Input: part model. Units: mm. Frame: model coordinates. Give positions to 0.01 mm unless a question says otherwise; leave off trailing zeros. Loops run counter-clockwise (first coordinate to the right, second up) from the corner with the lowest first, then second, coordinate; pieces in that order, holes last. Notation, with made-up numbers: (20.25, -36.75) - (29.25, -36.75) arc R20 ccw to (29.25, -29.75) - close; hole circle Ø11 at (50.25, 43). An arc over 180 degrees is marked (long way). Answer as a JSON object with one key per item and string values. Group by question number.
(1) Pin query (flat end, axial travel): P1, Ø4.5, axis at x = 60.325, z = -30.48, coming from the -Y side. Return the tip coordinate at first contact, or that it passes through.
(2) Section query D-D (z = 25.4). Return loops of the section in (x, y) (1 decimal), plus the area to 3 significant figures.
(3) Section query B-B (x = 0). Return loops of the section in (y, z), plus the area to 3 significant figures.
(4) Section query A-A (z = -30.48). Return loops of the section in (x, y) (3 decimals), plus the area to 3 significant figures.
(5) Mould query, pull axis Z, two halves, no side actions, for faces 1 (the flat face through (1, 2, 35.56)), 2 (the cylindrical face through (57.845, 2.129, -31.031)), 3 (the flat face through (66.675, 2, 0)). Classes: +Z half, -Z half, draft (parallel to the pull), parting line (faces both ways), or undercut.
(6) Section query C-C (z = 0). Return loops of the section in (x, y) (3 decimals), plus the area to 3 significant figures.
(7) Material intervals for L1, parallel to X at y = 3.15, z = 30.48 (3 decimals); L2, parallel to X at y = 3.6, z = -0.5 (3 decimals); L3, parallel to X at y = 1.25, z = 24.5 (3 decimals), sorted ascending.
```python
from build123d import *

# Parameters (mm, degrees)
SKETCH1_R           = 29.21
SKETCH1_R_2         = 2.2225
SKETCH1_R_3         = 2.54
BOSS_EXTRUDE1_DEPTH = 4.318


with BuildPart() as part:
    # Sketch1 → Boss-Extrude1 (new body)
    with BuildSketch(Plane(origin=(0, 0, 0), x_dir=(1, 0, 0), z_dir=(0, 1, 0))):
        Polygon((0, 35.56), (66.675, 35.56), (66.675, -35.56), (-66.675, -35.56), (-66.675, 35.56), align=None)
        with Locations(Location((0, 0, 0), (0, 0, 270))):
            Circle(SKETCH1_R, mode=Mode.SUBTRACT)
        with Locations(Location((25.4, -25.4, 0), (0, 0, 270))):
            Circle(SKETCH1_R_2, mode=Mode.SUBTRACT)
        with Locations(Location((25.4, 25.4, 0), (0, 0, 270))):
            Circle(SKETCH1_R_2, mode=Mode.SUBTRACT)
        with Locations(Location((-25.4, 25.4, 0), (0, 0, 270))):
            Circle(SKETCH1_R_2, mode=Mode.SUBTRACT)
        with Locations(Location((-25.4, -25.4, 0), (0, 0, 270))):
            Circle(SKETCH1_R_2, mode=Mode.SUBTRACT)
        with Locations(Location((-60.325, -30.48, 0), (0, 0, 270))):
            Circle(SKETCH1_R_3, mode=Mode.SUBTRACT)
        with Locations(Location((-60.325, 30.48, 0), (0, 0, 270))):
            Circle(SKETCH1_R_3, mode=Mode.SUBTRACT)
        with Locations(Location((60.325, 30.48, 0), (0, 0, 270))):
            Circle(SKETCH1_R_3, mode=Mode.SUBTRACT)
        with Locations(Location((60.325, -30.48, 0), (0, 0, 270))):
            Circle(SKETCH1_R_3, mode=Mode.SUBTRACT)
    extrude(amount=BOSS_EXTRUDE1_DEPTH)


solid = part.part
```
Recorded:
{
 "1": {"P1": "passes through"},
 "2": {"outline": "(-66.7, 0) - (-27.6, 0) - (-27.6, 4.3) - (-66.7, 4.3) - close; (-23.2, 0) - (-14.4, 0) - (-14.4, 4.3) - (-23.2, 4.3) - close; (14.4, 0) - (23.2, 0) - (23.2, 4.3) - (14.4, 4.3) - close; (27.6, 0) - (66.7, 0) - (66.7, 4.3) - (27.6, 4.3) - close", "area": "413 mm^2"},
 "3": {"outline": "(0, -35.56) - (4.32, -35.56) - (4.32, -29.21) - (0, -29.21) - close; (0, 29.21) - (4.32, 29.21) - (4.32, 35.56) - (0, 35.56) - close", "area": "54.8 mm^2"},
 "4": {"outline": "(-66.675, 0) - (-62.865, 0) - (-62.865, 4.318) - (-66.675, 4.318) - close; (-57.785, 0) - (57.785, 0) - (57.785, 4.318) - (-57.785, 4.318) - close; (62.865, 0) - (66.675, 0) - (66.675, 4.318) - (62.865, 4.318) - close", "area": "532 mm^2"},
 "5": {"face 1": "+Z half", "face 2": "undercut", "face 3": "draft"},
 "6": {"outline": "(-66.675, 0) - (-29.21, 0) - (-29.21, 4.318) - (-66.675, 4.318) - close; (29.21, 0) - (66.675, 0) - (66.675, 4.318) - (29.21, 4.318) - close", "area": "324 mm^2"},
 "7": {"L1": "x = -66.675 to -62.865, -57.785 to 57.785, 62.865 to 66.675", "L2": "x = -66.675 to -29.206, 29.206 to 66.675", "L3": "x = -66.675 to -27.432, -23.368 to -15.905, 15.905 to 23.368, 27.432 to 66.675"}
}
